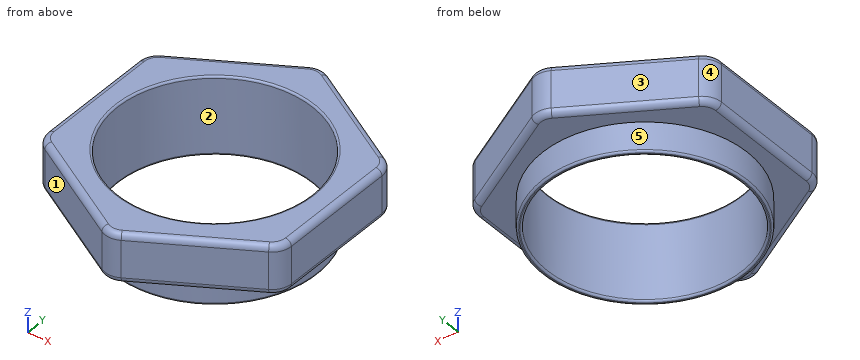
```python
from build123d import *

# Parameters (mm, degrees)
SKETCH1_R           = 6.6675
BOSS_EXTRUDE1_DEPTH = 1.905
BOSS_EXTRUDE2_DEPTH = 3.175
SKETCH3_R           = 6.35
CUT_EXTRUDE1_DEPTH  = 14.145931484
FILLET1_R           = 1.27
FILLET2_R           = 0.381
FILLET3_R           = 0.127


with BuildPart() as part:
    # Sketch1 → Boss-Extrude1 (new body)
    with BuildSketch(Plane.XY):
        with Locations(Location((0, 0, 0), (0, 0, 180))):
            Circle(SKETCH1_R)
    extrude(amount=BOSS_EXTRUDE1_DEPTH)

    # Sketch2 → Boss-Extrude2 (add)
    with BuildSketch(Plane.XY.offset(1.905)):
        Polygon((7.9375, 4.582717762), (0, 9.165435523), (-7.9375, 4.582717762), (-7.9375, -4.582717762), (0, -9.165435523), (7.9375, -4.582717762), align=None)
    extrude(amount=BOSS_EXTRUDE2_DEPTH)

    # Sketch3 → Cut-Extrude1 (cut, through all)
    with BuildSketch(Plane(origin=(0, 0, 0), x_dir=(-1, 0, 0), z_dir=(0, 0, -1))):
        Circle(SKETCH3_R)
    extrude(amount=-CUT_EXTRUDE1_DEPTH, mode=Mode.SUBTRACT)

    # Fillet1
    fillet1_edges = [part.edges().sort_by_distance(p)[0] for p in [
        (7.9375, 4.582717762, 3.4925),
        (0, 9.165435523, 3.4925),
        (-7.9375, 4.582717762, 3.4925),
        (-7.9375, -4.582717762, 3.4925),
        (0, -9.165435523, 3.4925),
        (7.9375, -4.582717762, 3.4925),
    ]]
    fillet(fillet1_edges, radius=FILLET1_R)

    # Fillet2
    fillet2_edges = [part.edges().sort_by_distance(p)[0] for p in [
        (3.96875, 6.874076643, 1.905),
        (3.96875, 6.874076643, 5.08),
        (7.9375, 0, 1.905),
        (3.96875, -6.874076643, 1.905),
        (-3.96875, -6.874076643, 1.905),
        (-7.9375, 0, 1.905),
        (-3.96875, 6.874076643, 1.905),
        (0, 8.96896584, 1.905),
        (-7.767352263, 4.48448292, 1.905),
        (-7.767352263, -4.48448292, 1.905),
        (0, -8.96896584, 1.905),
        (7.767352263, -4.48448292, 1.905),
        (7.767352263, 4.48448292, 1.905),
        (7.9375, 0, 5.08),
        (-3.96875, 6.874076643, 5.08),
        (-7.9375, 0, 5.08),
        (-3.96875, -6.874076643, 5.08),
        (3.96875, -6.874076643, 5.08),
        (0, 8.96896584, 5.08),
        (-7.767352263, 4.48448292, 5.08),
        (-7.767352263, -4.48448292, 5.08),
        (0, -8.96896584, 5.08),
        (7.767352263, -4.48448292, 5.08),
        (7.767352263, 4.48448292, 5.08),
    ]]
    fillet(fillet2_edges, radius=FILLET2_R)

    # Fillet3
    fillet3_edges = [part.edges().sort_by_distance(p)[0] for p in [
        (6.6675, 0, 0),
        (6.35, 0, 5.08),
        (6.35, 0, 0),
    ]]
    fillet(fillet3_edges, radius=FILLET3_R)


solid = part.part
```
Read the model definition and answer for the solid it produces. Units are mm, in the model's axes. Face numbers are marked on the shaded views. A direction names the side the tool comes from. Coordinates: 2 decimals unless noted, no trailing zeros. Answer as a JSON object with one key per item and string values. Group by question number.
Item 1: The mould has two halves that part along Y. Classify the marked faces 1, 2 and 3: +Y half, -Y half, draft (parallel to the pull), parting line (faces both ways), or undercut.
Item 2: Consider probe 1 along Y at (x, z) = (0, 2.3); probe 2 along Y at (x, z) = (0, 2); probe 3 along X at (y, z) = (-4.75, 1.3). Determine where each line is inside the solid, lowest interval first. Write a range as from..to.
Item 3: A flat-ended cylindrical pin translates along its axis: P1, Ø1.5, axis at x = -1, z = 1, coming from the +Y side. Find the tip coordinate at first contact, or state that the pin passes through.
Item 4: A tool of negligible diameter and unlimited length cuts with its end or side. For the marked faces 4 and 5, from which of +Z, -Z, +X, -X, +Y, -Y can it reach the whole face along a straight path? Write none if from no direction.
Results are:
{
 "1": {"face 1": "-Y half", "face 2": "undercut", "face 3": "+Y half"},
 "2": {"probe 1": "y = -8.97..-6.35, 6.35..8.97", "probe 2": "y = -8.84..-6.35, 6.35..8.84", "probe 3": "x = -4.68..-4.21, 4.21..4.68"},
 "3": {"P1": "stops at y = 6.66"},
 "4": {"face 4": "+Z, -Z, -X, +Y", "face 5": "-Z"}
}
